```python
from build123d import *


with BuildPart() as part:
    # Çizim1 → Döndür1 (revolve)
    with BuildSketch(Plane(origin=(0, 0, 0), x_dir=(0, 0, -1), z_dir=(1, 0, 0)), mode=Mode.PRIVATE) as d_nd_r1_sk:
        Polygon((-2.5, 15), (0, 8.964466094), (2.5, 15), (5, 15), (5, 5.63), (-5, 5.63), (-5, 15), align=None)
    revolve(d_nd_r1_sk.sketch.rotate(Axis((0, 0, 13.198807947), (0, 0, -1)), 90), axis=Axis((0, 0, 13.198807947), (0, 0, -1)))


solid = part.part
```
Check sheet for the modelled part. Datum: model origin and axes. Units: mm. A direction names the side the tool comes from. Give positions to 0.01 mm unless a question says otherwise; leave off trailing zeros. Order: outer loops, then holes, each group sorted by start corner. A loop starts at its lowest first (then second) coordinate and runs counter-clockwise, first axis right, second up. Notation, with made-up numbers: (-30.75, 68) -> (12.25, 68) arc R19 cw to (12.25, 79) -> close; hole circle Ø7 at (1, -9). An arc over 180 degrees is marked (long way). Return JSON: item names as keys, results as strings.
1. Material ranges on probe 1 along Y at (x, z) = (0, -3); probe 2 along Z at (x, y) = (-1.25, -13.5); probe 3 along Y at (x, z) = (0, -2), recorded low to high. Write a range as [from, to].
From the geometry:
{"probe 1": "[-15, -5.63], [5.63, 15]", "probe 2": "[-5, -1.9], [1.9, 5]", "probe 3": "[-13.79, -5.63], [5.63, 13.79]"}
2. Go/stop test with flat-tipped pins: P1, Ø6, axis at y = 9, z = 0, coming from the +X side; P2, Ø2, axis at x = 2, z = 1, coming from the -Y side; P3, Ø2, axis at x = 5, z = 3.5, coming from the -Y side. Record where each tip stops, or that it passes through.
From the geometry:
{"P1": "x = 13.08", "P2": "y = -13.65", "P3": "y = -14.46"}
3. Cross-section at A-A, the plane y = 0. Record the cut outline in (x, z), plus the area to 3 significant figures.
From the geometry:
{"outline": "(-15, -5) -> (-5.63, -5) -> (-5.63, 5) -> (-15, 5) -> (-15, 2.5) -> (-8.96, 0) -> (-15, -2.5) -> close; (5.63, -5) -> (15, -5) -> (15, -2.5) -> (8.96, 0) -> (15, 2.5) -> (15, 5) -> (5.63, 5) -> close", "area": "157 mm^2"}
4. Cross-section at C-C, the plane z = 4.25. Record the cut outline in (x, y).
From the geometry:
{"outline": "circle Ø30 at (0, 0); hole circle Ø11.26 at (0, 0)"}
5. Cross-section at D-D, the plane z = -1.25. Record the cut outline in (x, y), plus the area to 3 significant figures.
From the geometry:
{"outline": "circle Ø23.96 at (0, 0); hole circle Ø11.26 at (0, 0)", "area": "351 mm^2"}
6. Mould release check, pull along Y, two halves, no side actions. Record for faces 3 (the flat face through (0, 6, -5)), 4 (the cylindrical face through (-0.733, -5.582, 0.07)), 5 (the cylindrical face through (8.06, -12.65, -3.77)): +Y half, -Y half, draft (parallel to the pull), parting line (faces both ways), or undercut.
From the geometry:
{"face 3": "draft", "face 4": "undercut", "face 5": "parting line"}
7. Set-up check for faces 1 (the conical face through (-2.025, 9.12, -0.156)), 2 (the flat face through (-6, 0, 5)): record each of +Z, -Z, +X, -X, +Y, -Y from which the full face is reachable in a straight line by a thin tool's end or side.
From the geometry:
{"face 1": "none", "face 2": "+Z, +X, -X, +Y, -Y"}
